Input: dimensioned drawing with shaded views. Units: mm. Origin: part minimum x, y, z. Round coordinates to 2 decimals unless told otherwise and drop trailing zeros. Loops run counter-clockwise (first coordinate to the right, second up) from the corner with the lowest first, then second, coordinate; pieces in that order, holes last.
1) Section A-A, the plane y = 0.8. Return loops of the section in (x, z).
2) Section B-B, the plane x = 51. Return loops of the section in (y, z).
3) Section C-C, the plane z = 14. Return loops of the section in (x, y).
4) Ray query, line 1 along X through (y, z) = (0.85, 14); line 2 along X through (y, z) = (0.5, 12.5); line 3 along Z through (x, y) = (36, 0.8). Return the intervals inside material, ascending.
5) First-contact query: pin 1 (7 mm diameter, centred on x = 10, z = 14, fed in from +Y). Flat tip, straight axial feed; report the tip coordinate or a pass-through.
6) Section D-D, the plane z = 6. Return loops of the section in (x, y).
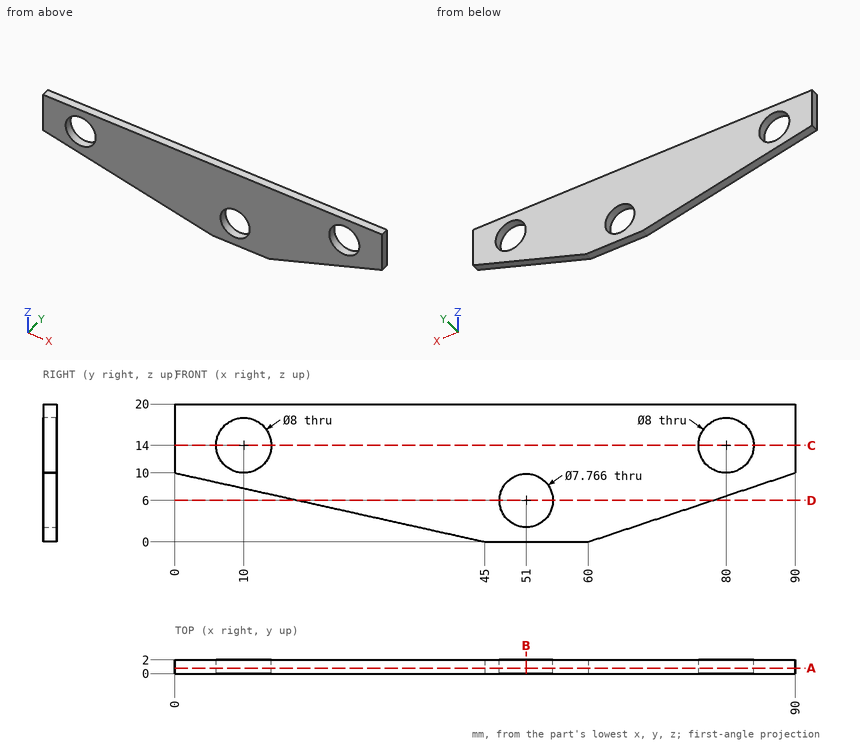
Final values:
1. outline: (0, 10) - (45, 0) - (60, 0) - (90, 10) - (90, 20) - (0, 20) - close; hole circle Ø8 at (10, 14); hole circle Ø7.77 at (51, 6); hole circle Ø8 at (80, 14)
2. outline: (0, 0) - (2, 0) - (2, 2.12) - (0, 2.12) - close; (0, 9.88) - (2, 9.88) - (2, 20) - (0, 20) - close
3. outline: (0, 0) - (6, 0) - (6, 2) - (0, 2) - close; (14, 0) - (76, 0) - (76, 2) - (14, 2) - close; (84, 0) - (90, 0) - (90, 2) - (84, 2) - close
4. line 1: x = 0 to 6, 14 to 76, 84 to 90
4. line 2: x = 0 to 6.29, 13.71 to 76.29, 83.71 to 90
4. line 3: z = 2 to 20
5. pin 1: passes through
6. outline: (18, 0) - (47.12, 0) - (47.12, 2) - (18, 2) - close; (54.88, 0) - (78, 0) - (78, 2) - (54.88, 2) - close
